from build123d import *

# Parameters (mm, degrees)
BOSS_EXTRUDE1_DEPTH     = 24.13
CUT_EXTRUDE1_DEPTH      = 139.595056638
CUT_EXTRUDE1_DEPTH_BACK = 139.595056638
FILLET1_R               = 1.5875
CUT_EXTRUDE2_DEPTH      = 12.7
CUT_EXTRUDE3_DEPTH      = 139.595056638
CUT_EXTRUDE3_DEPTH_BACK = 139.595056638
SKETCH4_R               = 3.2639
SHELL1_START            = -18.073116
SHELL1_DEPTH            = 36.146232
SHELL1_START_2          = -5.373116
SHELL1_2_DEPTH          = 10.746232


# Read off the part's stored shape, not the designer's step: Shell1
with BuildPart() as part:
    # Sketch1 → Boss-Extrude1 (new, symmetric)
    with BuildSketch(Plane.XY):
        with BuildLine():
            Line((56.161313585, 65.087564001), (56.15, 65.087371974))
            ThreePointArc((56.15, 65.087371974), (55.438759683, 64.766920639), (55.174115771, 64.033084522))
            Line((55.174115771, 64.033084522), (56.680450554, 36.457041128))
            ThreePointArc((56.680450554, 36.457041128), (56.705496383, 35.550244887), (56.681639728, 34.643416582))
            Line((56.681639728, 34.643416582), (55.144848554, 5.815734008))
            ThreePointArc((55.144848554, 5.815734008), (55.417746823, 5.074471658), (56.143430652, 4.7625))
            Line((56.143430652, 4.7625), (56.149999968, 4.762499984))
            ThreePointArc((56.149999968, 4.762499984), (56.857106771, 4.469606766), (57.15, 3.762499968))
            Line((57.15, 3.762499968), (57.15, -10.112499968))
            ThreePointArc((57.15, -10.112499968), (56.857106771, -10.819606766), (56.149999968, -11.112499984))
            Line((56.149999968, -11.112499984), (55.190522202, -11.1125))
            ThreePointArc((55.190522202, -11.1125), (54.502493828, -11.386816202), (54.191940103, -12.059266056))
            Line((54.191940103, -12.059266056), (53.961494186, -16.382053603))
            ThreePointArc((53.961494186, -16.382053603), (52.407837698, -21.109352316), (48.682296217, -24.408070592))
            Line((48.682296217, -24.408070592), (19.327486058, -38.967689038))
            ThreePointArc((19.327486058, -38.967689038), (0, -43.4975), (-19.327486058, -38.967689038))
            Line((-19.327486058, -38.967689038), (-19.327486058, -47.388950103))
            Line((-19.327486058, -47.388950103), (65.278, -47.388950103))
            Line((65.278, -47.388950103), (65.278, 119.854559949))
            Line((65.278, 119.854559949), (-4.702524006, 119.854559949))
            Line((-4.702524006, 119.854559949), (-4.702524006, 108.02491605))
            ThreePointArc((-4.702524006, 108.02491605), (0, 108.7374), (4.702524006, 108.02491605))
            Line((4.702524006, 108.02491605), (47.271514403, 94.82250963))
            ThreePointArc((47.271514403, 94.82250963), (51.961130003, 91.582350175), (53.960821068, 86.244526329))
            Line((53.960821068, 86.244526329), (54.197705155, 81.907956584))
            ThreePointArc((54.197705155, 81.907956584), (54.508664182, 81.236365226), (55.196216585, 80.9625))
            Line((55.196216585, 80.9625), (56.149999984, 80.962499984))
            ThreePointArc((56.149999984, 80.962499984), (56.857106777, 80.669606761), (57.15, 79.962499968))
            Line((57.15, 79.962499968), (57.15, 66.087500032))
            ThreePointArc((57.15, 66.087500032), (56.8610955, 65.384404568), (56.161313585, 65.087564001))
        make_face()
    extrude(amount=BOSS_EXTRUDE1_DEPTH, both=True)

    # Sketch2 → Cut-Extrude1 (cut, two sides: drawn at the far end of the back side and taken through both)
    with BuildSketch(Plane.XY.offset(-CUT_EXTRUDE1_DEPTH_BACK)):
        Polygon((0, 0), (16.649604997, 137.747881839), (-33.336773011, 132.313158031), (-32.126746787, -67.704176811), (15.765326083, -67.704176811), align=None)
    extrude(amount=CUT_EXTRUDE1_DEPTH + CUT_EXTRUDE1_DEPTH_BACK, mode=Mode.SUBTRACT)

    # Fillet1
    fillet1_edges = [part.edges().sort_by_distance(p)[0] for p in [
        (65.278, 119.854559949, 0),
        (65.278, -47.388950103, 0),
        (11.034802966, -47.388950103, 0),
        (9.864742858, -42.364128158, 0),
        (12.755119811, 105.527472687, 0),
        (14.486836775, 119.854559949, 0),
    ]]
    fillet(fillet1_edges, radius=FILLET1_R)

    # Sketch3 → Cut-Extrude2 (cut)
    with BuildSketch(Plane(origin=(0, 0, -24.13), x_dir=(-1, 0, 0), z_dir=(0, 0, -1))):
        Polygon((-39.878, -30.708992794), (-46.2788, -34.404496397), (-46.2788, -41.795503603), (-39.878, -45.491007206), (-33.4772, -41.795503603), (-33.4772, -34.404496397), align=None)
        Polygon((-33.4772, 111.645503603), (-39.878, 115.341007206), (-46.2788, 111.645503603), (-46.2788, 104.254496397), (-39.878, 100.558992794), (-33.4772, 104.254496397), align=None)
    cut_extrude2 = extrude(amount=-CUT_EXTRUDE2_DEPTH, mode=Mode.SUBTRACT)

    # Mirror1: Cut-Extrude2 across plane
    add(cut_extrude2.mirror(Plane.XY), mode=Mode.SUBTRACT)

    # Sketch4 → Cut-Extrude3 (cut, two sides: drawn at the far end of the back side and taken through both)
    with BuildSketch(Plane.XY.offset(-CUT_EXTRUDE3_DEPTH_BACK)):
        with Locations((39.878, 107.95)):
            Circle(SKETCH4_R)
        with Locations((39.878, -38.1)):
            Circle(SKETCH4_R)
    extrude(amount=CUT_EXTRUDE3_DEPTH + CUT_EXTRUDE3_DEPTH_BACK, mode=Mode.SUBTRACT)

    # Shell1 outline → Shell1 (cut)
    with BuildSketch(Plane.XY.offset(SHELL1_START)):
        Polygon((19.374447508, 109.816041015), (27.420316, 107.32068407), (27.420316, 115.142447211), (35.581934673, 119.854559949), (20.587804641, 119.854559949), align=None)
        with BuildLine():
            Line((52.335684, 100.757552789), (50.881166896, 99.917786948))
            ThreePointArc((50.881166896, 99.917786948), (57.51024809, 94.223530979), (60.031332227, 85.856129752))
            ThreePointArc((60.031332227, 85.856129752), (62.362476281, 83.309849707), (63.206884, 79.962499968))
            Line((63.206884, 79.962499968), (63.206884008, 66.087500032))
            ThreePointArc((63.206884008, 66.087500032), (62.736011515, 63.552926254), (61.386232226, 61.356592716))
            Line((61.386232226, 61.356592716), (62.728318266, 36.787404457))
            ThreePointArc((62.728318266, 36.787404457), (62.762379081, 35.55421632), (62.729935471, 34.320984576))
            Line((62.729935471, 34.320984576), (61.354914269, 8.527841436))
            ThreePointArc((61.354914269, 8.527841436), (62.727616894, 6.318780038), (63.206884, 3.762499968))
            Line((63.206884, 3.762499968), (63.206884, -10.112499968))
            ThreePointArc((63.206884, -10.112499968), (62.362476281, -13.459849707), (60.031332227, -16.006129752))
            ThreePointArc((60.031332227, -16.006129752), (57.656879346, -24.143823794), (51.373585166, -29.834193295))
            Line((51.373585166, -29.834193295), (50.891079569, -30.073510032))
            Line((50.891079569, -30.073510032), (52.335684, -30.907552789))
            Line((52.335684, -30.907552789), (52.335684, -45.292447211))
            Line((52.335684, -45.292447211), (48.704434473, -47.388950103))
            Line((48.704434473, -47.388950103), (63.6905, -47.388950103))
            ThreePointArc((63.6905, -47.388950103), (64.813032015, -46.923982118), (65.278, -45.801450103))
            Line((65.278, -45.801450103), (65.278, 118.267059949))
            ThreePointArc((65.278, 118.267059949), (64.813032015, 119.389591964), (63.6905, 119.854559949))
            Line((63.6905, 119.854559949), (44.174065327, 119.854559949))
            Line((44.174065327, 119.854559949), (52.335684, 115.142447211))
            Line((52.335684, 115.142447211), (52.335684, 100.757552789))
        make_face()
        with BuildLine():
            Line((17.253727402, -47.388950103), (31.051565527, -47.388950103))
            Line((31.051565527, -47.388950103), (27.420316, -45.292447211))
            Line((27.420316, -45.292447211), (27.420316, -41.714715011))
            Line((27.420316, -41.714715011), (22.018775007, -44.39381174))
            ThreePointArc((22.018775007, -44.39381174), (19.565089882, -45.528499114), (17.053178169, -46.527691625))
            Line((17.053178169, -46.527691625), (17.253727402, -47.388950103))
        make_face()
    extrude(amount=SHELL1_DEPTH, mode=Mode.SUBTRACT)

    # Shell1 2 outline → Shell1 2 (cut)
    with BuildSketch(Plane.XY.offset(SHELL1_START_2)):
        with BuildLine():
            Line((31.051565527, -47.388950103), (39.108311519, -47.388950103))
            ThreePointArc((39.108311519, -47.388950103), (33.724832418, -45.101110132), (30.764746274, -40.055919453))
            Line((30.764746274, -40.055919453), (27.420316, -41.714715011))
            Line((27.420316, -41.714715011), (27.420316, -45.292447211))
            Line((27.420316, -45.292447211), (31.051565527, -47.388950103))
        make_face()
        with BuildLine():
            ThreePointArc((30.704014451, 106.302273224), (42.639021135, 116.852459024), (46.509623897, 101.40029933))
            Line((46.509623897, 101.40029933), (49.065696603, 100.607555354))
            ThreePointArc((49.065696603, 100.607555354), (49.984188595, 100.290983166), (50.881166896, 99.917786948))
            Line((50.881166896, 99.917786948), (52.335684, 100.757552789))
            Line((52.335684, 100.757552789), (52.335684, 115.142447211))
            Line((52.335684, 115.142447211), (44.174065327, 119.854559949))
            Line((44.174065327, 119.854559949), (35.581934673, 119.854559949))
            Line((35.581934673, 119.854559949), (27.420316, 115.142447211))
            Line((27.420316, 115.142447211), (27.420316, 107.32068407))
            Line((27.420316, 107.32068407), (30.704014451, 106.302273224))
        make_face()
        with BuildLine():
            Line((40.647688481, -47.388950103), (48.704434473, -47.388950103))
            Line((48.704434473, -47.388950103), (52.335684, -45.292447211))
            Line((52.335684, -45.292447211), (52.335684, -30.907552789))
            Line((52.335684, -30.907552789), (50.891079569, -30.073510032))
            Line((50.891079569, -30.073510032), (46.949876749, -32.028297304))
            ThreePointArc((46.949876749, -32.028297304), (48.501221551, -41.637946362), (40.647688481, -47.388950103))
        make_face()
    extrude(amount=SHELL1_2_DEPTH, mode=Mode.SUBTRACT)


solid = part.part
The listing builds one solid part. Answer for the finished solid, in the listing's coordinates (mm). A direction names the side the tool comes from. Round coordinates to 2 decimals unless told otherwise and drop trailing zeros. Order: outer loops, then holes, each group sorted by start corner. A loop starts at its lowest first (then second) coordinate and runs counter-clockwise, first axis right, second up. Notation, with made-up numbers: (17, 7) -> (51, 7) arc R32 ccw to (51, 34) -> close; hole circle Ø11 at (88, 47.25). An arc over 180 degrees is marked (long way). Put each result on its own line as item: value.
Q1. Section C-C, the plane y = 42.5 is taken. Write down the section's boundary in (x, z).
Results list:
outline: (56.35, -24.13) -> (65.28, -24.13) -> (65.28, -18.07) -> (62.42, -18.07) -> (62.42, 18.07) -> (65.28, 18.07) -> (65.28, 24.13) -> (56.35, 24.13) -> close
Q2. Determine the mould class of faces 6 (the flat face through (27.42, 111, 12)), 7 (the flat face through (58, 43, 24.13)), 8 (the cylindrical face through (39.453, 111.186, -0.16)) for opening direction Z: pulls with the +Z half, pulls with the -Z half, needs draft (parallel to the pull), parting line crosses it, or undercut.
Results list:
face 6: undercut
face 7: pulls with the +Z half
face 8: needs draft
Q3. Section B-B, the plane z = 9 is taken. Count the separate pieces of the cut face and the enclosed holes in it, and give its area (3 significant figures).
Results list:
separate pieces: 1
enclosed holes: 2
area: 1,950 mm^2
Q4. Section A-A, the plane y = 68.5 is taken. Write down the section's boundary in (x, z), and give its area (3 significant figures).
Results list:
outline: (57.15, -24.13) -> (65.28, -24.13) -> (65.28, -18.07) -> (63.21, -18.07) -> (63.21, 18.07) -> (65.28, 18.07) -> (65.28, 24.13) -> (57.15, 24.13) -> close
area: 317 mm^2
Q5. Consider line 1 along Y through (x, z) = (35, 16); line 2 along Y through (x, z) = (42, -6); line 3 along Y through (x, z) = (14.5, -11). Determine where each line is inside the solid, lowest interval first.
Results list:
line 1: -47.39 to -42.67, -33.53 to -31.19, 98.63 to 103.38, 112.52 to 119.52
line 2: -47.39 to -40.58, -35.62 to -27.72, 96.46 to 105.47, 110.43 to 119.85
line 3: -47.39 to -41.01, 104.99 to 119.03
Q6. Which of the six approach directions +Z, -Z, +X, -X, +Y, -Y give full straight-line access (tool end or side, diameter ignored) to faces 1 (the flat face through (36.72, 102.38, 17.87)), 2 (the flat face through (64, 37, 18.073)), 3 (the cylindrical face through (15.469, -40.654, 0.338)), 4 (the flat face through (36.633, 113.467, -17.869)), 5 (the flat face through (50.545, -46.326, 11.634))?
Results list:
face 1: +Z
face 2: +X
face 3: +Z, -Z, -X
face 4: -Z
face 5: +X, -Y
Q7. Each of these flat-tipped pins is pushed along its axis until it touches: P1, Ø4, axis at y = -5.5, z = -2.5, coming from the +X side; P2, Ø1, axis at y = 37.5, z = -2, coming from the +X side; P3, Ø6.5, axis at y = 107.5, z = -12.5, coming from the +X side; P4, Ø12, axis at x = 49, y = 15.5, coming from the -Z side. Where does it stop, or does it pass through?
Results list:
P1: x = 63.21
P2: x = 62.72
P3: x = 52.34
P4: through
